The model under review builds one solid part; all positions refer to its coordinate system, in mm. Round coordinates to 2 decimals unless told otherwise and drop trailing zeros. Write each loop counter-clockwise with the first axis right and the second up, starting at its lowest first coordinate (ties: lowest second). Pieces come first, ordered by that corner, then holes. Notation, with made-up numbers: (79, 78.5) -> (96, 78.5) arc R21 cw to (96, 95.5) -> close; hole circle Ø4 at (18.5, 9). An arc over 180 degrees is marked (long way). Answer as a JSON object with one key per item and string values. Group by question number.
1) We need section C-C, the plane z = 14. Write out the cut boundary in (x, y).
2) We need section A-A, the plane y = 0. Write out the cut boundary in (x, z) (3 decimals).
3) Mouldability with a two-part tool opening along Y and no side actions: class faces 1 (the flat face through (-35.242, 0, 9)), 2 (the flat face through (0, 22.542, 9)), 3 (the cylindrical face through (-34.518, -21.779, 9.336)), 4 (the cylindrical face through (-0.83, -3.72, 9.34)) as pulls with the +Y half, pulls with the -Y half, needs draft (parallel to the pull), parting line crosses it, or undercut.
4) To check wall thickness, follow probe 1 along Y at (x, z) = (0, 10.25); probe 2 along X at (y, z) = (-1, 15.5); probe 3 along X at (y, z) = (3, 1.75). State the ranges of each line that lie inside material, in increasing order. Write a range as [from, to].
5) We need section B-B, the plane x = 0. Write out the cut boundary in (y, z) (1 decimal), then the cut area to 3 significant figures.
from build123d import *

# Parameters (mm, degrees)
SKETCH2_W           = 70.484
SKETCH2_H           = 45.085
BOSS_EXTRUDE1_DEPTH = 18.415
FILLET1_R           = 2.54
SKETCH3_R           = 3.81
CUT_EXTRUDE1_DEPTH  = 46.708588856


with BuildPart() as part:
    # Sketch2 → Boss-Extrude1 (new body)
    with BuildSketch(Plane.XY):
        Rectangle(SKETCH2_W, SKETCH2_H)
    extrude(amount=BOSS_EXTRUDE1_DEPTH)

    # Fillet1
    fillet1_edges = [part.edges().sort_by_distance(p)[0] for p in [
        (35.242, -22.5425, 9.2075),
        (-35.242, -22.5425, 9.2075),
        (-35.242, 22.5425, 9.2075),
        (35.242, 22.5425, 9.2075),
    ]]
    fillet(fillet1_edges, radius=FILLET1_R)

    # Sketch3 → Cut-Extrude1 (cut, through all)
    with BuildSketch(Plane.XY.offset(18.415)):
        Circle(SKETCH3_R)
    extrude(amount=-CUT_EXTRUDE1_DEPTH, mode=Mode.SUBTRACT)


solid = part.part
Here are the results:
{
 "1": {"outline": "(-35.24, -20) arc R2.54 ccw to (-32.7, -22.54) -> (32.7, -22.54) arc R2.54 ccw to (35.24, -20) -> (35.24, 20) arc R2.54 ccw to (32.7, 22.54) -> (-32.7, 22.54) arc R2.54 ccw to (-35.24, 20) -> close; hole circle Ø7.62 at (0, 0)"},
 "2": {"outline": "(-35.242, 0) -> (-3.81, 0) -> (-3.81, 18.415) -> (-35.242, 18.415) -> close; (3.81, 0) -> (35.242, 0) -> (35.242, 18.415) -> (3.81, 18.415) -> close"},
 "3": {"face 1": "needs draft", "face 2": "pulls with the +Y half", "face 3": "pulls with the -Y half", "face 4": "undercut"},
 "4": {"probe 1": "y = [-22.54, -3.81], [3.81, 22.54]", "probe 2": "x = [-35.24, -3.68], [3.68, 35.24]", "probe 3": "x = [-35.24, -2.35], [2.35, 35.24]"},
 "5": {"outline": "(-22.5, 0) -> (-3.8, 0) -> (-3.8, 18.4) -> (-22.5, 18.4) -> close; (3.8, 0) -> (22.5, 0) -> (22.5, 18.4) -> (3.8, 18.4) -> close", "area": "690 mm^2"}
}
